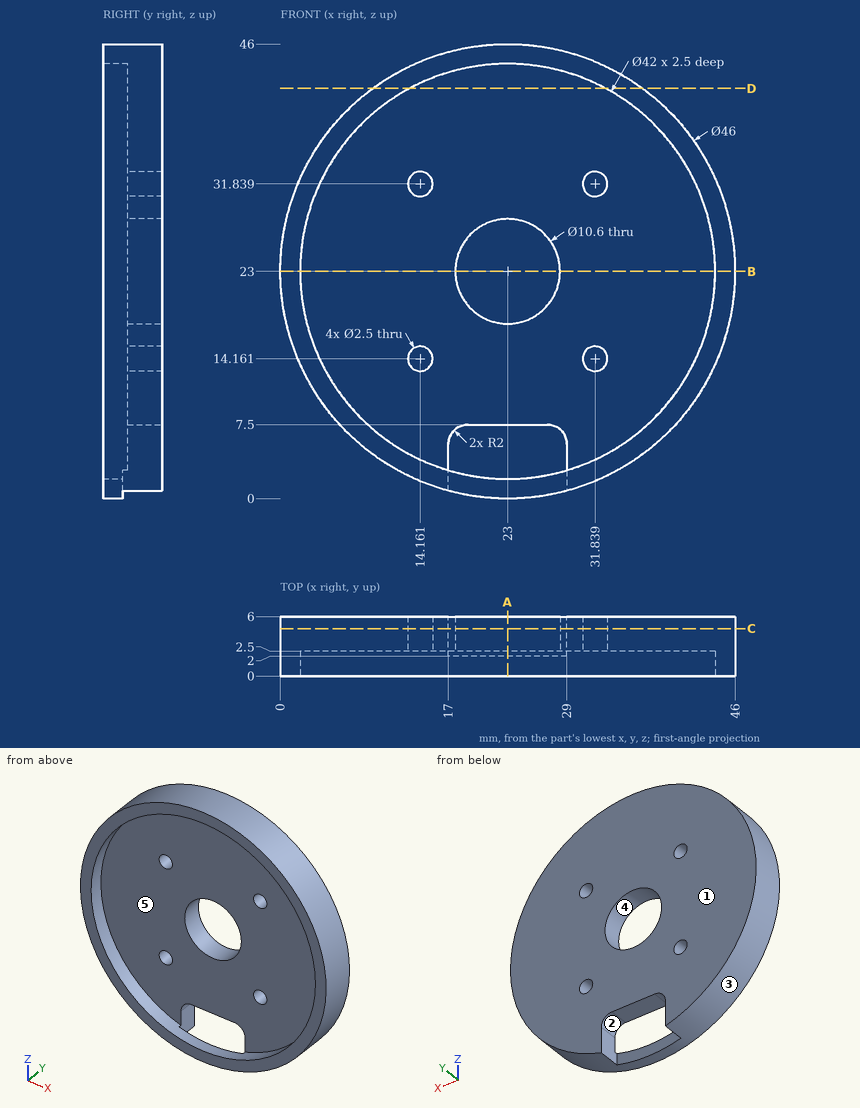
The figure shows three views and two pictorial views of one solid part (mm, origin at its lowest corner). Answer the questions. A direction names the side the tool comes from. Round coordinates to 2 decimals unless told otherwise and drop trailing zeros. Loops run counter-clockwise (first coordinate to the right, second up) from the corner with the lowest first, then second, coordinate; pieces in that order, holes last. Notation, with made-up numbers: (81.25, -3.75) - (129.25, -3.75) arc R11 ccw to (129.25, 1.25) - close; hole circle Ø1 at (30, 62.5). An arc over 180 degrees is marked (long way). Use one line per item in the form item = value. Start each with the question number.
(1) Consider line 1 (X direction, y = 5.3, z = 23); line 2 (X direction, y = 2.9, z = 13.5); line 3 (Z direction, x = 23, y = 1.3). Determine where each line is inside the solid, lowest interval first.
(2) Find section D-D on z = 41.5. Determine the outline of the cut face in (x, y).
(3) Which of the six approach directions +Z, -Z, +X, -X, +Y, -Y give full straight-line access (tool end or side, diameter ignored) to the marked faces 4 and 5?
(4) Find section C-C on y = 4.8. Determine the outline of the cut face in (x, z), and give its area (3 significant figures).
(5) Determine the mould class of the marked faces 1, 2 and 3 for opening direction X: +X half, -X half, draft (parallel to the pull), parting line (faces both ways), or undercut.
(6) Find section B-B on z = 23. Determine the outline of the cut face in (x, y), and give its area (3 significant figures).
(7) Flat-ended cylindrical pins translate along their axes: P1, Ø17, axis at x = 23, z = 23, coming from the +Y side; P2, Ø3, axis at x = 31.84, z = 14.16, coming from the -Y side; P3, Ø1.8, axis at x = 21.5, y = 4, coming from the -Z side; P4, Ø2, axis at x = 29.5, y = 2.5, coming from the +Z side. Find the tip coordinate at first contact, or state that the pin passes through.
(8) Find section A-A on x = 23. Determine the outline of the cut face in (y, z), and give its area (3 significant figures).
Answer list:
q1.line_1 = 0 to 17.7, 28.3 to 46
q1.line_2 = 2.05 to 13.1, 15.22 to 30.78, 32.9 to 43.95
q1.line_3 = 0 to 2, 44 to 46
q2.outline = (9.33, 0) - (13.06, 0) - (13.06, 2.5) - (32.94, 2.5) - (32.94, 0) - (36.67, 0) - (36.67, 6) - (9.33, 6) - close
q3.face_4 = +Y, -Y
q3.face_5 = -Y
q4.outline = (17, 0.8) - (17, 5.5) arc R2 cw to (19, 7.5) - (27, 7.5) arc R2 cw to (29, 5.5) - (29, 0.8) arc R23 ccw (long way) to start; hole circle Ø2.5 at (14.16, 14.16); hole circle Ø2.5 at (14.16, 31.84); hole circle Ø10.6 at (23, 23); hole circle Ø2.5 at (31.84, 14.16); hole circle Ø2.5 at (31.84, 31.84)
q4.area = 1,470 mm^2
q5.face_1 = draft
q5.face_2 = undercut
q5.face_3 = parting line
q6.outline = (0, 0) - (2, 0) - (2, 2.5) - (17.7, 2.5) - (17.7, 6) - (0, 6) - close; (28.3, 2.5) - (44, 2.5) - (44, 0) - (46, 0) - (46, 6) - (28.3, 6) - close
q6.area = 134 mm^2
q7.P1 = 6
q7.P2 = 2.5
q7.P3 = 7.5
q7.P4 = 45.33
q8.outline = (0, 0) - (2, 0) - (2, 2) - (0, 2) - close; (0, 44) - (2.5, 44) - (2.5, 28.3) - (6, 28.3) - (6, 46) - (0, 46) - close; (2.5, 7.5) - (6, 7.5) - (6, 17.7) - (2.5, 17.7) - close
q8.area = 107 mm^2
